Check sheet for the modelled part. Datum: model origin and axes. Units: mm. Face numbers are marked on the shaded views. A direction names the side the tool comes from. Coordinates: 2 decimals unless noted, no trailing zeros. Loops run counter-clockwise (first coordinate to the right, second up) from the corner with the lowest first, then second, coordinate; pieces in that order, holes last. Notation, with made-up numbers: M 28.25,46 L 87.25,46 A29 ccw 87.25,78 Z; hole C 63.25,18.25 d4. An arc over 180 degrees is marked long. Use CSV: the item, a comma, the result in double quotes. Start each with the question number.
(1) Set-up check for the marked faces 4, 5 and 6: record each of +Z, -Z, +X, -X, +Y, -Y from which the full face is reachable in a straight line by a thin tool's end or side.
(2) Go/stop test with flat-tipped pins: pin 1 Ø4.5 at (y, z) = (-16, 3.5) entering from +X; pin 2 Ø4.5 at (x, z) = (-4.5, 3.5) entering from +Y; pin 3 Ø3 at (x, y) = (-5, -15.18) entering from -Z; pin 4 Ø6 at (x, z) = (10.5, 2) entering from +Y. Record where each tip stops, or that it passes through.
(3) Draft check along X on the marked faces 1, 2 and 3. Enter one of: pulls with the +X half, pulls with the -X half, needs draft (parallel to the pull), parting line crosses it, or undercut.
(4) Scan lines: line 1 (X direction, y = -15.18, z = 7.75); line 2 (X direction, y = -14, z = 5.25); line 3 (Y direction, x = -5, z = 6.5). Record each from-to range of solid material in increasing order.
(5) Section check D-D on x = 1.5. Record the cut outline in (y, z), and give its area (3 significant figures).
(6) Section check A-A on y = -15.18. Record the cut outline in (x, z).
(7) Section check C-C on z = 4. Give the number of separate pieces and of enclosed holes in the cut face, and give its area (3 significant figures).
(8) Section check B-B on x = -5. Record the cut outline in (y, z).
from build123d import *

# Parameters (mm, degrees)
F1_DEPTH = 10
F2_D     = 3.3
F3_SIZE  = 0.5
F4_R     = 0.5
F5_SIZE  = 0.5


with BuildPart() as f1:
    # F0 (on Top) → F1 (new body)
    with BuildSketch(Plane.XY):
        Polygon((9.75, -9.43), (21.035, 6.69), (21.035, 19.43), (19.0360967857, 19.43), (18.035, 14.42), (12.745, 14.42), (12.745, 13.22), (-14.835, 13.22), (-14.835, 16.93), (-18.035, 16.93), (-18.5345492942, 19.43), (-21.035, 19.43), (-21.035, 6.69), (-9.75, -9.43), (-9.75, -19.43), (9.75, -19.43), align=None)
    extrude(amount=F1_DEPTH)

    # F2 (through all)
    with Locations(Plane(origin=(0, 0, 0), x_dir=(1, 0, 0), z_dir=(0, 0, -1))):
        with Locations((5, 15.18), (-5, 15.18)):
            Hole(F2_D / 2)

    # F3
    f3_edges = [f1.edges().sort_by_distance(p)[0] for p in [
        (-15.3925, -1.37, 10),
        (-21.035, 13.06, 10),
        (-9.75, -14.43, 10),
        (-19.784775, 19.43, 10),
        (0, -19.43, 10),
        (-18.284775, 18.18, 10),
        (9.75, -14.43, 10),
        (-16.435, 16.93, 10),
        (15.3925, -1.37, 10),
        (-14.835, 15.075, 10),
        (21.035, 13.06, 10),
        (-1.045, 13.22, 10),
        (20.035548, 19.43, 10),
        (12.745, 13.82, 10),
        (18.535548, 16.925, 10),
        (15.39, 14.42, 10),
        (-6.65, -15.18, 10),
        (3.35, -15.18, 10),
        (-15.3925, -1.37, 0),
        (-21.035, 13.06, 0),
        (-9.75, -14.43, 0),
        (-19.784775, 19.43, 0),
        (0, -19.43, 0),
        (-18.284775, 18.18, 0),
        (9.75, -14.43, 0),
        (-16.435, 16.93, 0),
        (15.3925, -1.37, 0),
        (-14.835, 15.075, 0),
        (21.035, 13.06, 0),
        (-1.045, 13.22, 0),
        (20.035548, 19.43, 0),
        (12.745, 13.82, 0),
        (18.535548, 16.925, 0),
        (15.39, 14.42, 0),
        (-6.65, -15.18, 0),
        (3.35, -15.18, 0),
    ]]
    chamfer(f3_edges, length=F3_SIZE)

    # F4
    f4_edges = [f1.edges().sort_by_distance(p)[0] for p in [
        (-21.035, 19.43, 5),
        (-18.534549, 19.43, 5),
        (-18.035, 16.93, 5),
        (-14.835, 16.93, 5),
        (-14.835, 13.22, 5),
        (21.035, 19.43, 5),
        (19.036097, 19.43, 5),
        (18.035, 14.42, 5),
        (12.745, 14.42, 5),
        (12.745, 13.22, 5),
    ]]
    fillet(f4_edges, radius=F4_R)

    # F5
    f5_edges = [f1.edges().sort_by_distance(p)[0] for p in [
        (-9.75, -19.43, 5),
        (9.75, -19.43, 5),
    ]]
    chamfer(f5_edges, length=F5_SIZE)


solid = f1.part
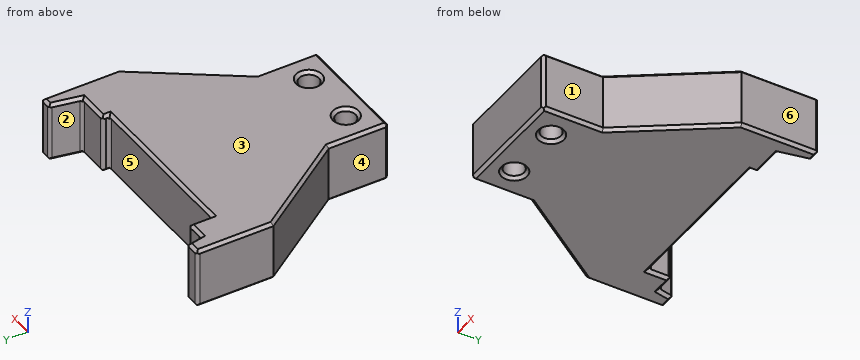
Outcome:
1,face 4,"+Z, -Z, -X, -Y"
1,face 5,"+Z, -Z, +Y"
1,face 6,"+Z, -Z, +X, +Y, -Y"
2,pin 1,"stops at x = 9.75"
2,pin 2,"stops at y = 13.22"
2,pin 3,"passes through"
2,pin 4,"stops at y = 14.42"
3,face 1,"pulls with the +X half"
3,face 2,"undercut"
3,face 3,"needs draft"
4,line 1,"x = -9.75 to -6.65, -3.35 to 3.35, 6.65 to 9.75"
4,line 2,"x = -9.75 to -6.15, -3.85 to 3.85, 6.15 to 9.75"
4,line 3,"y = -19.43 to -16.83, -13.53 to 13.22"
5,outline,"M -19.43,0.5 L -18.93,0 L 12.72,0 L 13.22,0.5 L 13.22,9.5 L 12.72,10 L -18.93,10 L -19.43,9.5 Z"
5,area,"326 mm²"
6,outline,"M -9.75,0.5 L -9.25,0 L -7.15,0 L -6.65,0.5 L -6.65,9.5 L -7.15,10 L -9.25,10 L -9.75,9.5 Z; M -3.35,0.5 L -2.85,0 L 2.85,0 L 3.35,0.5 L 3.35,9.5 L 2.85,10 L -2.85,10 L -3.35,9.5 Z; M 6.65,0.5 L 7.15,0 L 9.25,0 L 9.75,0.5 L 9.75,9.5 L 9.25,10 L 7.15,10 L 6.65,9.5 Z"
7,separate pieces,"1"
7,enclosed holes,"2"
7,area,"1,000 mm²"
8,outline,"M -19.43,0.5 L -18.93,0 L -17.33,0 L -16.83,0.5 L -16.83,9.5 L -17.33,10 L -18.93,10 L -19.43,9.5 Z; M -13.53,0.5 L -13.03,0 L 12.72,0 L 13.22,0.5 L 13.22,9.5 L 12.72,10 L -13.03,10 L -13.53,9.5 Z"
